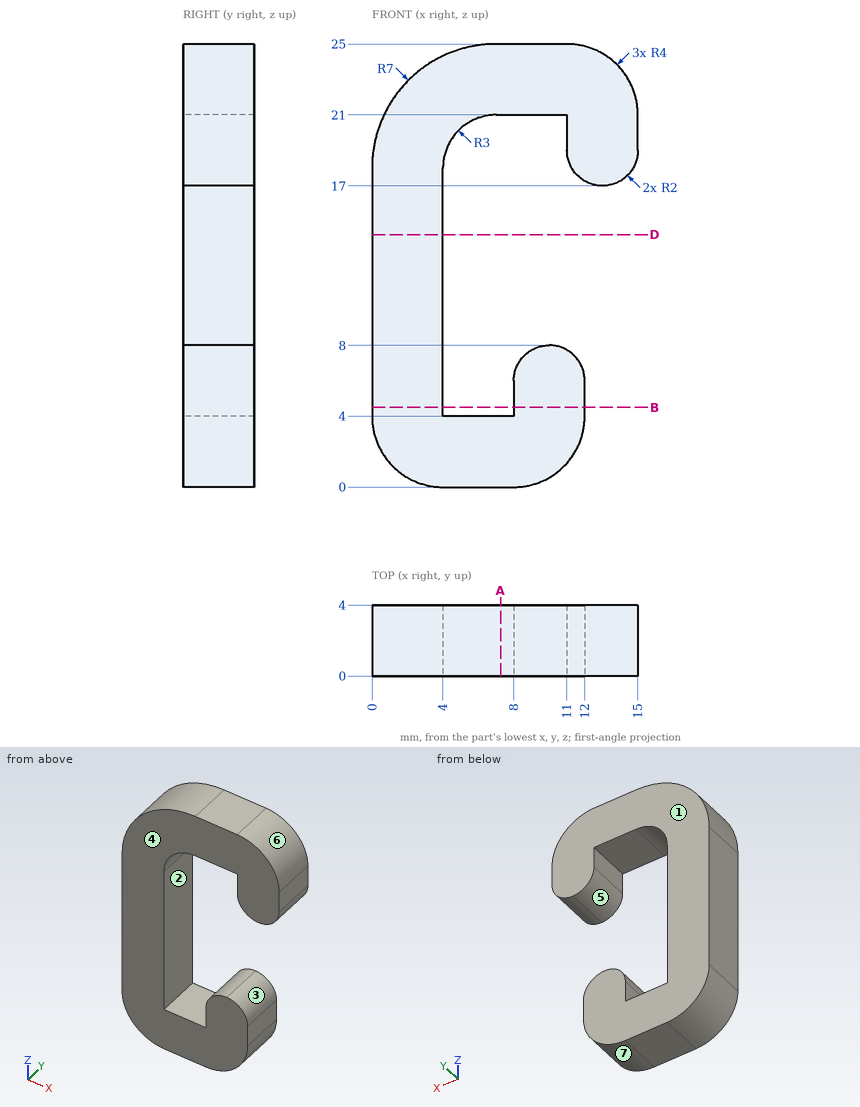
Study the drawing (mm; zero at the part's minimum x, y, z) and answer. A direction names the side the tool comes from. Round coordinates to 2 decimals unless told otherwise and drop trailing zeros. Order: outer loops, then holes, each group sorted by start corner. A loop starts at its lowest first (then second) coordinate and runs counter-clockwise, first axis right, second up. Notation, with made-up numbers: M 74.25,19 L 127.25,19 A10 ccw 127.25,37 Z; hole C -26,23 d7. An arc over 180 degrees is marked long. One line per item, written item: value.
Q1. Find section B-B on z = 4.5. Write down the section's boundary in (x, y).
Derived:
outline: M 0,0 L 4,0 L 4,4 L 0,4 Z; M 8,0 L 12,0 L 12,4 L 8,4 Z
Q2. For the marked faces 1, 2 and 3, determine the directions among +Z, -Z, +X, -X, +Y, -Y from which every point of the face is accessible in a straight line to the end or side of a thin tool.
Derived:
face 1: +Z, -Z, +X, -X, +Y
face 2: +Y, -Y
face 3: +X, +Y, -Y
Q3. Straight lines are drawn through the part: line 1 (X direction, y = 0.5, z = 8.25); line 2 (Z direction, x = 7, y = 2.25); line 3 (Z direction, x = 8.25, y = 3.4). For each, find the intervals that lie inside material, in ascending order.
Derived:
line 1: 0 to 4
line 2: 0 to 4, 21 to 25
line 3: 0.01 to 6.97, 21 to 25
Q4. Find section A-A on x = 7.25. Write down the section's boundary in (y, z).
Derived:
outline: M 0,0 L 4,0 L 4,4 L 0,4 Z; M 0,21 L 4,21 L 4,25 L 0,25 Z
Q5. Flat-ended cylindrical pins translate along their axes: pin 1 (2 mm diameter, centred on y = 2, z = 5, fed in from +X); pin 2 (1.6 mm diameter, centred on y = 1.5, z = 20, fed in from -X); pin 3 (1.2 mm diameter, centred on y = 1.5, z = 13.5, fed in from +X); pin 4 (1 mm diameter, centred on y = 1, z = 5.5, fed in from -X). Find the tip coordinate at first contact, or state that the pin passes through.
Derived:
pin 1: x = 12
pin 2: x = 0.1
pin 3: x = 4
pin 4: x = 0
Q6. Find section D-D on z = 14.25. Write down the section's boundary in (x, y).
Derived:
outline: M 0,0 L 4,0 L 4,4 L 0,4 Z
Q7. Determine the mould class of the marked faces 4, 5, 6 and 7 for opening direction Z: released by +Z, released by -Z, zero draft, split by the parting line, or undercut.
Derived:
face 4: zero draft
face 5: undercut
face 6: released by +Z
face 7: released by -Z
